Source: CAD feature listing. Evaluate the final solid. Frame: model axes, mm. Face numbers are marked on the shaded views. Give positions to 0.01 mm unless a question says otherwise; leave off trailing zeros. Order: outer loops, then holes, each group sorted by start corner. A loop starts at its lowest first (then second) coordinate and runs counter-clockwise, first axis right, second up. Notation, with made-up numbers: (-34.5, 46.25) - (-1.5, 46.25) arc R23 ccw to (-1.5, 81.25) - close; hole circle Ø11 at (86, 14.25). An arc over 180 degrees is marked (long way). Answer as CSV lines item,"result".
Autodesk Inventor part; units mm, degrees
ref_plane "YZ Plane" through (0, 0, 0) normal (1, 0, 0) x (0, 1, 0)
ref_plane "XZ Plane" through (0, 0, 0) normal (0, 1, 0) x (-1, 0, 0)
ref_plane "XY Plane" through (0, 0, 0) normal (0, 0, 1) x (1, 0, 0)
sketch "Sketch1" plane through (0, 0, 0) normal (0, 1, 0) x (-1, 0, 0)
  line L0 (750, -375) -> (-750, -375)
  line L1 (-750, -375) -> (-750, 375)
  line L2 (-750, 375) -> (750, 375)
  line L3 (750, 375) -> (750, -375)
  line L4 (0, 0) -> (-250, 0) construction
  line L5 (0, 0) -> (0, -250) construction
  dimension "d0" = 1500
  dimension "d1" = 750
  dimension "d2" = 250
  dimension "d3" = 250
extrude "Extrusion1" add sketch "Sketch1" along normal blind 40
fillet "Fillet1" radius 10 4 edges at (750, 20, 375) (750, 20, -375) (-750, 20, -375) (-750, 20, 375)
fillet "Fillet2" radius 5 8 edges at (-747.0711, 40, -372.0711) (-750, 40, 0) (-747.0711, 40, 372.0711) (0, 40, 375) (747.0711, 40, 372.0711) (750, 40, 0) (747.0711, 40, -372.0711) (0, 40, -375)
sketch "Sketch2" plane through (0, 0, 0) normal (0, -1, 0) x (1, 0, 0)
  line L0 (0, 0) -> (400, 0) construction
  line L1 (750, -365) -> (750, 365) construction
  line L2 (300, 200) -> (500, 200)
  line L3 (500, 200) -> (500, -200)
  line L4 (500, -200) -> (300, -200)
  line L5 (300, -200) -> (300, 200)
  line L6 (400, 0) -> (400, -100) construction
  line L7 (0, 0) -> (0, 100) construction
  line L8 (-300, 200) -> (-500, 200)
  line L9 (-500, 200) -> (-500, -200)
  line L10 (-500, -200) -> (-300, -200)
  line L11 (-300, -200) -> (-300, 200)
  dimension "d8" = 400
  dimension "d10" = 200
  dimension "d11" = 400
  dimension "d14" = 100
  dimension "d15" = 100
extrude "Extrusion2" add sketch "Sketch2" along normal blind 10
sketch "Sketch3" plane through (0, -10, 0) normal (0, -1, 0) x (1, 0, 0)
  line L0 (0, 0) -> (400, 0) construction
  line L1 (400, 0) -> (400, 100) construction
  line L2 (362.5, -37.5) -> (437.5, -37.5)
  line L3 (437.5, -37.5) -> (437.5, 37.5)
  line L4 (437.5, 37.5) -> (362.5, 37.5)
  line L5 (362.5, 37.5) -> (362.5, -37.5)
  line L6 (0, 0) -> (0, 100) construction
  line L7 (-362.5, -37.5) -> (-437.5, -37.5)
  line L8 (-437.5, -37.5) -> (-437.5, 37.5)
  line L9 (-437.5, 37.5) -> (-362.5, 37.5)
  line L10 (-362.5, 37.5) -> (-362.5, -37.5)
  dimension "d18" = 400
  dimension "d19" = 100
  dimension "d20" = 75
  dimension "d21" = 75
  dimension "d22" = 100
extrude "Extrusion3" add sketch "Sketch3" along normal blind 500
sketch "Sketch4" plane through (0, -510, 0) normal (0, -1, 0) x (1, 0, 0)
  line L0 (0, 0) -> (400, 0) construction
  line L1 (400, 0) -> (400, 100) construction
  line L2 (400, 0) -> (400, -100) construction
  line L3 (350, 200) -> (450, 200)
  line L4 (450, 200) -> (450, -200)
  line L5 (450, -200) -> (350, -200)
  line L6 (350, -200) -> (350, 200)
  line L7 (0, 0) -> (0, 100) construction
  line L8 (-350, 200) -> (-450, 200)
  line L9 (-450, 200) -> (-450, -200)
  line L10 (-450, -200) -> (-350, -200)
  line L11 (-350, -200) -> (-350, 200)
  dimension "d25" = 400
  dimension "d26" = 100
  dimension "d27" = 100
  dimension "d28" = 100
  dimension "d29" = 400
  dimension "d30" = 100
extrude "Extrusion4" add sketch "Sketch4" along normal blind 50
fillet "Fillet3" radius 5 8 edges at (437.5, -260, -37.5) (362.5, -260, -37.5) (437.5, -260, 37.5) (-362.5, -260, -37.5) (-362.5, -260, 37.5) (-437.5, -260, -37.5) (362.5, -260, 37.5) (-437.5, -260, 37.5)
fillet "Fillet4" radius 5 12 edges at (-400, -510, 200) (-450, -535, 200) (-350, -535, 200) (350, -535, 200) (400, -510, 200) (450, -535, 200) (350, -535, -200) (-450, -535, -200) (-400, -510, -200) (-350, -535, -200) (400, -510, -200) (450, -535, -200)
properties part number "Table"
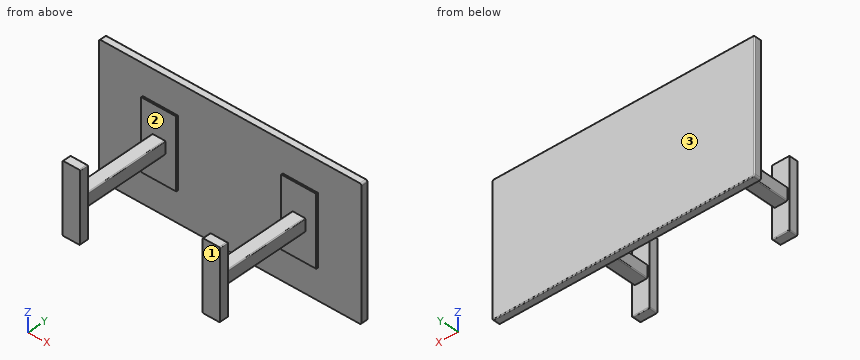
(1) Cut plane A-A (y = -113.5). Return loops of the section in (x, z), then the cut area to 3 significant figures.
Completed:
outline,"(-437.5, -32.5) arc R5 ccw to (-432.5, -37.5) - (-367.5, -37.5) arc R5 ccw to (-362.5, -32.5) - (-362.5, 32.5) arc R5 ccw to (-367.5, 37.5) - (-432.5, 37.5) arc R5 ccw to (-437.5, 32.5) - close; (362.5, -32.5) arc R5 ccw to (367.5, -37.5) - (432.5, -37.5) arc R5 ccw to (437.5, -32.5) - (437.5, 32.5) arc R5 ccw to (432.5, 37.5) - (367.5, 37.5) arc R5 ccw to (362.5, 32.5) - close"
area,"11,200 mm²"
(2) Cut plane C-C (x = 413.5). Return loops of the section in (y, z), then the cut area to 3 significant figures.
Completed:
outline,"(-560, -200) - (-515, -200) arc R5 ccw to (-510, -195) - (-510, -37.5) - (-10, -37.5) - (-10, -200) - (0, -200) - (0, -375) - (35, -375) arc R5 ccw to (40, -370) - (40, 370) arc R5 ccw to (35, 375) - (0, 375) - (0, 200) - (-10, 200) - (-10, 37.5) - (-510, 37.5) - (-510, 195) arc R5 ccw to (-515, 200) - (-560, 200) - close"
area,"91,500 mm²"
(3) Ray query, line 1 (X direction, y = -534.5, z = -85); line 2 (X direction, y = -348.5, z = -28.5); line 3 (Y direction, x = -149.5, z = 115). Return the intervals inside material, ascending. Write a range as from..to.
Completed:
line 1,"-450..-350, 350..450"
line 2,"-437.5..-362.5, 362.5..437.5"
line 3,"0..40"
(4) Cut plane B-B (z = -138.5). Return loops of the section in (x, y), then the cut area to 3 significant figures.
Completed:
outline,"(-750, 0) - (-500, 0) - (-500, -10) - (-300, -10) - (-300, 0) - (300, 0) - (300, -10) - (500, -10) - (500, 0) - (750, 0) - (750, 35) arc R5 ccw to (745, 40) - (-745, 40) arc R5 ccw to (-750, 35) - close; (-450, -560) - (-350, -560) - (-350, -510) - (-450, -510) - close; (350, -560) - (450, -560) - (450, -510) - (350, -510) - close"
area,"74,000 mm²"
(5) Contact query for flat-ended pins moving along their axis: pin 1 (3 mm diameter, centred on x = -448, y = -7, fed in from +Z); pin 2 (19.5 mm diameter, centred on x = 385.5, y = -200, fed in from -Z); pin 3 (15 mm diameter, centred on y = -535, z = 12.5, fed in from -X). Output: stop coordinate, or through.
Completed:
pin 1,"z = 200"
pin 2,"z = -37.5"
pin 3,"x = -450"
(6) Mould query, pull axis Y, two halves, no side actions, for the marked faces 1, 2 and 3. Classes: released by +Y, released by -Y, zero draft, split by the parting line, or undercut.
Completed:
face 1,"released by -Y"
face 2,"undercut"
face 3,"released by +Y"
(7) Cut plane D-D (z = 289). Return loops of the section in (x, y).
Completed:
outline,"(-750, 0) - (750, 0) - (750, 35) arc R5 ccw to (745, 40) - (-745, 40) arc R5 ccw to (-750, 35) - close"
